```python
from build123d import *

# Parameters (mm, degrees)
BOSS_EXTRUDE1_DEPTH     = 100
CUT_EXTRUDE3_DEPTH      = 550.891405391
CUT_EXTRUDE3_DEPTH_BACK = 550.891405391
CUT_EXTRUDE5_DEPTH      = 550.686535404
CUT_EXTRUDE5_DEPTH_BACK = 550.686535404


with BuildPart() as part:
    # Sketch1 → Boss-Extrude1 (new body)
    with BuildSketch(Plane.XY):
        with BuildLine():
            ThreePointArc((-192.629438793, 0), (-136.135725272, 33.719619965), (-73.991525193, 55.321722514))
            ThreePointArc((-73.991525193, 55.321722514), (231.264395529, 54.89097703), (535.785554592, 33.719619965))
            ThreePointArc((535.785554592, 33.719619965), (534.174229279, 3.332708678), (535.785554592, -27.054202608))
            ThreePointArc((535.785554592, -27.054202608), (235.762691459, -64.934671976), (-66.568309368, -71.614065728))
            ThreePointArc((-66.568309368, -71.614065728), (-137.800866021, -50.244872094), (-192.629438793, 0))
        make_face()
    extrude(amount=BOSS_EXTRUDE1_DEPTH)

    # Sketch2 → Cut-Extrude3 (cut, two sides: drawn at the far end of the back side and taken through both)
    with BuildSketch(Plane(origin=(0, 0, 0), x_dir=(0, 0, -1), z_dir=(1, 0, 0)).offset(-CUT_EXTRUDE3_DEPTH_BACK)):
        with BuildLine():
            ThreePointArc((-65.447202994, 54.830423707), (-80.892507985, 50.983746932), (-92.956496986, 40.600368972))
            ThreePointArc((-92.956496986, 40.600368972), (-98.736407831, -10.977338679), (-88.967303886, -61.950193259))
            ThreePointArc((-88.967303886, -61.950193259), (-83.10915251, -68.165990231), (-75.589128758, -72.216090516))
            ThreePointArc((-75.589128758, -72.216090516), (-123.822815089, -94.064788666), (-173.378544397, -75.407784602))
            ThreePointArc((-173.378544397, -75.407784602), (-163.802190068, -4.583325871), (-135.262897635, 60.940099743))
            ThreePointArc((-135.262897635, 60.940099743), (-100.366866686, 80.430667917), (-61.326949176, 89.003885783))
            ThreePointArc((-61.326949176, 89.003885783), (-63.560434952, 71.938056418), (-65.447202994, 54.830423707))
        make_face()
    extrude(amount=CUT_EXTRUDE3_DEPTH + CUT_EXTRUDE3_DEPTH_BACK, mode=Mode.SUBTRACT)

    # Sketch3 → Cut-Extrude5 (cut, two sides: drawn at the far end of the back side and taken through both)
    with BuildSketch(Plane(origin=(0, 0, 0), x_dir=(0, 0, -1), z_dir=(1, 0, 0)).offset(-CUT_EXTRUDE5_DEPTH_BACK)):
        with BuildLine():
            ThreePointArc((-74.208303325, 50.886642831), (-50.335012976, 52.211638999), (-26.713093985, 48.511024166))
            ThreePointArc((-26.713093985, 48.511024166), (-16.247111553, 43.841102683), (-7.714956491, 36.189482926))
            ThreePointArc((-7.714956491, 36.189482926), (-2.445034952, -12.786836037), (-8.678058045, -61.649923489))
            ThreePointArc((-8.678058045, -61.649923489), (-17.453523943, -70.69509128), (-29.511303704, -74.360307413))
            ThreePointArc((-29.511303704, -74.360307413), (33.955140221, -79.826327987), (85.286434054, -42.104117568))
            ThreePointArc((85.286434054, -42.104117568), (41.180066923, 16.064388488), (12.319514625, 83.116720583))
            ThreePointArc((12.319514625, 83.116720583), (-170.558095104, 441.821406771), (-74.208303325, 50.886642831))
        make_face()
    extrude(amount=CUT_EXTRUDE5_DEPTH + CUT_EXTRUDE5_DEPTH_BACK, mode=Mode.SUBTRACT)


solid = part.part
```
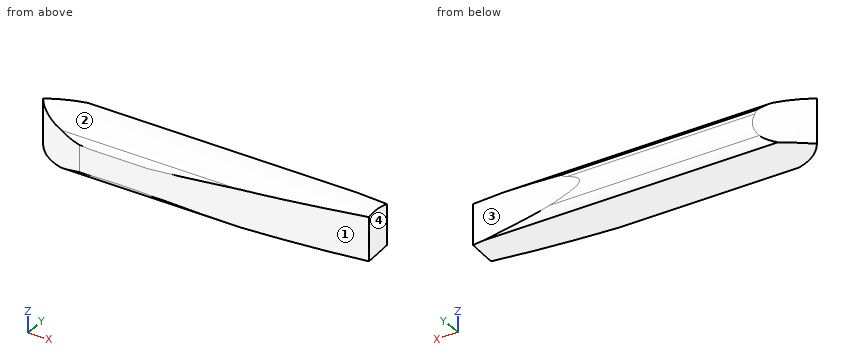
Could you check a few things on this model? Use its own coordinates, in mm. Face numbers are marked on the shaded views. Give positions to 0.01 mm unless a question says otherwise; leave off trailing zeros. Order: outer loops, then holes, each group sorted by start corner. A loop starts at its lowest first (then second) coordinate and runs counter-clockwise, first axis right, second up.
Q1. Suppose I cut it at B-B, the plane z = 33. Write out the boundary of the cut face in (x, y), and give its area (3 significant figures).
Q2. If I drill on line 1 along Z through (x, y) = (-122, -2); line 2 along X through (y, z) = (-15.5, 60.5); line 3 along Z through (x, y) = (210.5, 22.5), over which ranges is the centre line in solid material (lowest first)?
Q3. Suppose I cut it at D-D, the plane x = 487.5. Write out the boundary of the cut face in (y, z), and give its area (3 significant figures).
Q4. I'm going to push flat-ended pins straight in: P1, Ø6, axis at x = 230, y = 21, coming from the -Z side; P2, Ø12, axis at x = 187, y = -28.5, coming from the -Z side; P3, Ø2, axis at x = 251.5, y = -52, coming from the -Z side. Where does each tip first touch, or does it pass through?
Q5. We'd pull the mould along Y, two halves only. Please class the marked faces 1, 2, 3 and 4: +Y half, -Y half, draft (parallel to the pull), parting line (faces both ways), or undercut.
Q6. Suppose I cut it at A-A, the plane x = 310.5. Write out the boundary of the cut face in (y, z).
Solution:
1. outline: (-192.63, 0) arc R166.54 ccw to (-66.57, -71.61) arc R2922.96 ccw to (535.79, -27.05) arc R287.33 cw to (535.79, 33.72) arc R4489.88 ccw to (335.26, 50) - (-93.66, 50) arc R323.75 ccw to start
1. area: 74,900 mm2
2. line 1: z = 2.61 to 98.85
2. line 2: x = -180.53 to 534.79
2. line 3: z = 5.07 to 96.79
3. outline: (-35.29, 3.87) arc R210.93 ccw to (36.19, 7.71) arc R36.96 ccw to (38.47, 9.73) - (38.47, 93.51) arc R173.11 ccw to (-35.29, 96.06) - close
3. area: 6,900 mm2
4. P1: stops at z = 4.4
4. P2: stops at z = 2.76
4. P3: stops at z = 6.32
5. face 1: -Y half
5. face 2: parting line
5. face 3: +Y half
5. face 4: undercut
6. outline: (-58.44, 7.91) arc R210.93 ccw to (36.19, 7.71) arc R36.96 ccw to (48.51, 26.71) arc R113.61 ccw to (51.38, 41.19) - (51.38, 70.83) arc R113.61 ccw to (50.89, 74.21) arc R202.65 cw to (49.99, 82.69) arc R34.43 ccw to (40.6, 92.96) arc R173.11 ccw to (-58.44, 90.17) - close
